```python
from build123d import *

# Parameters (mm, degrees)
SKETCH_1_R          = 6
SKETCH_1_R_2        = 1.6
EXTRUDE_1_DEPTH     = 4
CUT_EXTRUDE_2_DEPTH = 71.329581259
FILLET_1_R          = 5


with BuildPart() as part:
    # 草图1 → 凸台-拉伸1 (new body)
    with BuildSketch(Plane(origin=(0, 0, 0), x_dir=(0, 0, -1), z_dir=(1, 0, 0))):
        with BuildLine():
            Line((-17.5, -47), (-17.5, -68))
            Line((-17.5, -68), (17.5, -68))
            Line((17.5, -68), (17.5, -47))
            Line((17.5, -47), (9.879034185, 1.550704218))
            ThreePointArc((9.879034185, 1.550704218), (0, 10), (-9.879034185, 1.550704218))
            Line((-9.879034185, 1.550704218), (-17.5, -47))
        make_face()
        Circle(SKETCH_1_R, mode=Mode.SUBTRACT)
        with Locations((-12.5, -50)):
            Circle(SKETCH_1_R_2, mode=Mode.SUBTRACT)
        with Locations((12.5, -50)):
            Circle(SKETCH_1_R_2, mode=Mode.SUBTRACT)
        with Locations((-12.5, -63)):
            Circle(SKETCH_1_R_2, mode=Mode.SUBTRACT)
        with Locations((12.5, -63)):
            Circle(SKETCH_1_R_2, mode=Mode.SUBTRACT)
    extrude(amount=EXTRUDE_1_DEPTH)

    # 草图3 → 切除-拉伸2 (cut, through all)
    with BuildSketch(Plane(origin=(4, 0, 0), x_dir=(0, 0, -1), z_dir=(1, 0, 0))):
        with BuildLine():
            Line((-6.920512772, -11.844929578), (-11.943527577, -43.844929578))
            ThreePointArc((-11.943527577, -43.844929578), (-11.715581533, -44.649972914), (-10.955624159, -45))
            Line((-10.955624159, -45), (10.955624159, -45))
            ThreePointArc((10.955624159, -45), (11.715581533, -44.649972914), (11.943527577, -43.844929578))
            Line((11.943527577, -43.844929578), (6.920512772, -11.844929578))
            ThreePointArc((6.920512772, -11.844929578), (6.582582268, -11.240042626), (5.932609354, -11))
            Line((5.932609354, -11), (-5.932609354, -11))
            ThreePointArc((-5.932609354, -11), (-6.582582268, -11.240042626), (-6.920512772, -11.844929578))
        make_face()
        with BuildLine():
            Line((-10.5, -55.196152423), (-10.5, -57.803847577))
            ThreePointArc((-10.5, -57.803847577), (-10.366025404, -58.303847577), (-10, -58.669872981))
            ThreePointArc((-10, -58.669872981), (-8.394106246, -60.146644697), (-7.569933514, -62.166666667))
            ThreePointArc((-7.569933514, -62.166666667), (-7.229417441, -62.763762616), (-6.583920217, -63))
            Line((-6.583920217, -63), (6.583920217, -63))
            ThreePointArc((6.583920217, -63), (7.229417441, -62.763762616), (7.569933514, -62.166666667))
            ThreePointArc((7.569933514, -62.166666667), (8.394106246, -60.146644697), (10, -58.669872981))
            ThreePointArc((10, -58.669872981), (10.366025404, -58.303847577), (10.5, -57.803847577))
            Line((10.5, -57.803847577), (10.5, -55.196152423))
            ThreePointArc((10.5, -55.196152423), (10.366025404, -54.696152423), (10, -54.330127019))
            ThreePointArc((10, -54.330127019), (8.394106246, -52.853355303), (7.569933514, -50.833333333))
            ThreePointArc((7.569933514, -50.833333333), (7.229417441, -50.236237384), (6.583920217, -50))
            Line((6.583920217, -50), (-6.583920217, -50))
            ThreePointArc((-6.583920217, -50), (-7.229417441, -50.236237384), (-7.569933514, -50.833333333))
            ThreePointArc((-7.569933514, -50.833333333), (-8.394106246, -52.853355303), (-10, -54.330127019))
            ThreePointArc((-10, -54.330127019), (-10.366025404, -54.696152423), (-10.5, -55.196152423))
        make_face()
    extrude(amount=-CUT_EXTRUDE_2_DEPTH, mode=Mode.SUBTRACT)

    # 圆角1
    fillet_1_edges = [part.edges().sort_by_distance(p)[0] for p in [
        (2, -47, -17.5),
        (2, -68, -17.5),
        (2, -68, 17.5),
        (2, -47, 17.5),
    ]]
    fillet(fillet_1_edges, radius=FILLET_1_R)


solid = part.part
```
The listing builds one solid part. Answer for the finished solid, in the listing's coordinates (mm). A direction names the side the tool comes from. Coordinates: 2 decimals unless noted, no trailing zeros. Loops run counter-clockwise (first coordinate to the right, second up) from the corner with the lowest first, then second, coordinate; pieces in that order, holes last. Notation, with made-up numbers: (10, 6.5) - (60, 6.5) arc R22 ccw to (60, 28.5) - close; hole circle Ø11 at (12.25, 61). An arc over 180 degrees is marked (long way). Write item = value, one per line.
1) Which of the six approach directions +Z, -Z, +X, -X, +Y, -Y give full straight-line access (tool end or side, diameter ignored) to faces 1 (the face through (2, -56, 10.5)), 2 (the face through (4, -46, 0))?
Responses:
face_1 = +X, -X
face_2 = +Z, -Z, +X, +Y, -Y
2) Section B-B (y = -59.5) is taken. Determine the outline of the cut face in (x, z), plus the area to 3 significant figures.
Responses:
outline = (0, -17.5) - (4, -17.5) - (4, -8.93) - (0, -8.93) - close; (0, 8.93) - (4, 8.93) - (4, 17.5) - (0, 17.5) - close
area = 68.6 mm^2
3) Each of these flat-tipped pins is pushed along its axis until it touches: P1, Ø8, axis at y = -45, z = -4, coming from the -X side; P2, Ø6, axis at y = -25.5, z = 4, coming from the +X side; P3, Ø1.2, axis at x = 3, z = -2, coming from the +Y side. Where does it stop, or does it pass through?
Responses:
P1 = 0
P2 = through
P3 = 9.9
4) Find the intervals of material crossed by line 1 along Z through (x, y) = (3.2, -57); line 2 along Z through (x, y) = (1, -62.5); line 3 along Z through (x, y) = (3.6, -38), in increasing order.
Responses:
line_1 = -17.5 to -10.5, 10.5 to 17.5
line_2 = -17.5 to -14.02, -10.98 to -7.45, 7.45 to 10.98, 14.02 to 17.5
line_3 = -16.09 to -11.03, 11.03 to 16.09
5) Section D-D (y = 0) is taken. Determine the outline of the cut face in (x, z).
Responses:
outline = (0, -10.12) - (4, -10.12) - (4, -6) - (0, -6) - close; (0, 6) - (4, 6) - (4, 10.12) - (0, 10.12) - close
6) Section A-A (z = 0) is taken. Determine the outline of the cut face in (x, y), plus the area to 3 significant figures.
Responses:
outline = (0, -68) - (4, -68) - (4, -63) - (0, -63) - close; (0, -50) - (4, -50) - (4, -45) - (0, -45) - close; (0, -11) - (4, -11) - (4, -6) - (0, -6) - close; (0, 6) - (4, 6) - (4, 10) - (0, 10) - close
area = 76.0 mm^2
7) Determine the mould class of faces 3 (the face through (2, -68, 0)), 4 (the face through (2, -55, -17.5)), 5 (the face through (2.028, -60.121, 8.412)), 6 (the face through (2, -45, 0)) for opening direction Y: pulls with the +Y half, pulls with the -Y half, needs draft (parallel to the pull), parting line crosses it, or undercut.
Responses:
face_3 = pulls with the -Y half
face_4 = needs draft
face_5 = undercut
face_6 = undercut
8) Section C-C (x = 1.2) is taken. Count the separate pieces of the cut face and the enclosed holes in it, plus the area to 3 significant figures.
Responses:
separate_pieces = 1
enclosed_holes = 7
area = 1,160 mm^2
